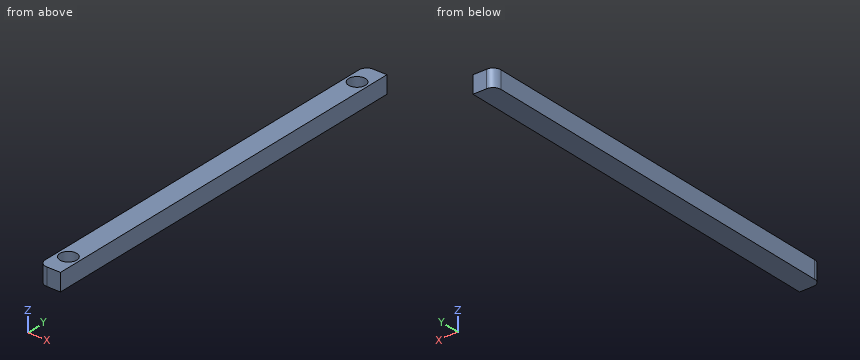
from build123d import *

# Parameters (mm, degrees)
SKETCH010_W  = 75.9
SKETCH010_H  = 3.301254
PAD004_DEPTH = 4.1
SKETCH_R     = 1.6
POCKET_DEPTH = 2.2
FILLET_R     = 1.5


with BuildPart() as part:
    # Sketch010 → Pad004 (new body)
    with BuildSketch(Plane.YZ):
        with Locations((-37.95, 12.349373)):
            Rectangle(SKETCH010_W, SKETCH010_H)
    extrude(amount=-PAD004_DEPTH)

    # Sketch (on Face4 of Pad004) → Pocket (cut)
    with BuildSketch(Plane(origin=(0, 0, 14), x_dir=(0, -1, 0), z_dir=(0, 0, 1))):
        with Locations((4.45, -2.05)):
            Circle(SKETCH_R)
        with Locations((71.55, -2.05)):
            Circle(SKETCH_R)
    extrude(amount=-POCKET_DEPTH, mode=Mode.SUBTRACT)

    # Fillet
    fillet_edges = [part.edges().sort_by_distance(p)[0] for p in [
        (-4.1, -75.9, 12.349373),
        (-4.1, 0, 12.349373),
    ]]
    fillet(fillet_edges, radius=FILLET_R)


solid = part.part
The listing builds one solid part. Answer for the finished solid, in the listing's coordinates (mm). Give positions to 0.01 mm unless a question says otherwise; leave off trailing zeros. Loops run counter-clockwise (first coordinate to the right, second up) from the corner with the lowest first, then second, coordinate; pieces in that order, holes last. Notation, with made-up numbers: M 56,85 L 103,85 A20 cw 103,94 Z; hole C -15,-24.5 d8. An arc over 180 degrees is marked long. Answer as CSV lines item,"result".
Item 1: Straight lines are drawn through the part: line 1 along X through (y, z) = (-71.55, 12.8); line 2 along Y through (x, z) = (-1.9, 12.1); line 3 along Y through (x, z) = (-1.3, 13.55). For each, find the intervals that lie inside material, in ascending order. Write a range as [from, to].
Values follow:
line 1,"x = [-4.1, -3.65], [-0.45, 0]"
line 2,"y = [-75.9, -73.14], [-69.96, -6.04], [-2.86, 0]"
line 3,"y = [-75.9, -72.96], [-70.14, -5.86], [-3.04, 0]"
Item 2: The part is cut by section A-A (z = 12.7). Give the vertices of the cut face in (x, y), and give its area (3 significant figures).
Values follow:
outline,"M -4.1,-74.4 A1.5 ccw -2.6,-75.9 L 0,-75.9 L 0,0 L -2.6,0 A1.5 ccw -4.1,-1.5 Z; hole C -2.05,-71.55 d3.2; hole C -2.05,-4.45 d3.2"
area,"294 mm^2"
Item 3: The part is cut by section B-B (y = -71.55). Give the vertices of the cut face in (x, z), and give its area (3 significant figures).
Values follow:
outline,"M -4.1,10.7 L 0,10.7 L 0,14 L -0.45,14 L -0.45,11.8 L -3.65,11.8 L -3.65,14 L -4.1,14 Z"
area,"6.50 mm^2"
Item 4: Given pin 1 Ø1 at (x, y) = (-1.5, -5) entering from +Z, flat-ended and moving along its own axis, determine where the tip first touches the part or whether it passes through.
Values follow:
pin 1,"stops at z = 11.8"
